Here's how the part is built. I have some questions about the finished solid (model axes, mm). Face numbers are marked on the shaded views. A direction names the side the tool comes from. Round coordinates to 2 decimals unless told otherwise and drop trailing zeros. Loops run counter-clockwise (first coordinate to the right, second up) from the corner with the lowest first, then second, coordinate; pieces in that order, holes last. Notation, with made-up numbers: M 45,-29.75 L 101,-29.75 A25 ccw 101,7.25 Z; hole C 2,9.25 d8. An arc over 180 degrees is marked long. Answer as a JSON object with one key per item and string values.
Solid Edge part; units mm, degrees
sketch "Sketch1" plane through (0, 0, 0) normal (0, -1, 0) x (1, 0, 0)
  line L0 (38.1517, 0) -> (38.1517, -10)
  line L1 (38.1517, -10) -> (28.1517, -10)
  line L2 (28.1517, -10) -> (28.1517, -20)
  line L3 (28.1517, -20) -> (38.1517, -20)
  line L4 (38.1517, -20) -> (38.1517, -46)
  line L5 (38.1517, -46) -> (28.1517, -46)
  line L6 (28.1517, -46) -> (28.1517, -56)
  line L7 (-21.8483, -56) -> (28.1517, -56)
  line L8 (-21.8483, -46) -> (-21.8483, -56)
  line L9 (-31.8483, -46) -> (-21.8483, -46)
  line L10 (-31.8483, -20) -> (-31.8483, -46)
  line L11 (-21.8483, -20) -> (-31.8483, -20)
  line L12 (-21.8483, -10) -> (-21.8483, -20)
  line L13 (-31.8483, -10) -> (-21.8483, -10)
  line L14 (-31.8483, 0) -> (-31.8483, -10)
  line L15 (-36.8483, 0) -> (-31.8483, 0)
  line L16 (-36.8483, 37) -> (-36.8483, 0)
  line L17 (-36.8483, 37) -> (43.1517, 37)
  line L18 (43.1517, 37) -> (43.1517, 0)
  line L19 (38.1517, 0) -> (43.1517, 0)
extrude "Extrusionsausprägung_1" add sketch "Sketch1" against normal blind 5 and the other way blind 0.001
sketch "Sketch2" plane through (3.1517, 5, -9.5) normal (0, 1, 0) x (0, 0, -1)
  line L0 (-46.5, 40) -> (-22.5, 40)
  line L1 (-22.5, 40) -> (-22.5, -40)
  line L2 (-22.5, -40) -> (-48.5, -40)
  line L3 (-48.5, -40) -> (-48.5, 40)
  line L4 (-48.5, 40) -> (-46.5, 40)
extrude "Extrusionsausprägung_2" add sketch "Sketch2" along normal blind 5 and the other way blind 0.001
sketch "Sketch3" plane through (43.1517, 4.9995, 19.5) normal (1, 0, 0) x (0, 0, -1)
  line L0 (-19.5, 5.0005) -> (6.5, 0.0005)
  line L1 (6.5, 0.0005) -> (9.9801, 7.8832)
  line L2 (9.9801, 7.8832) -> (-19.5, 5.0005)
extrude "Extrusionsausschnitt_1" cut sketch "Sketch3" against normal blind 96.3179
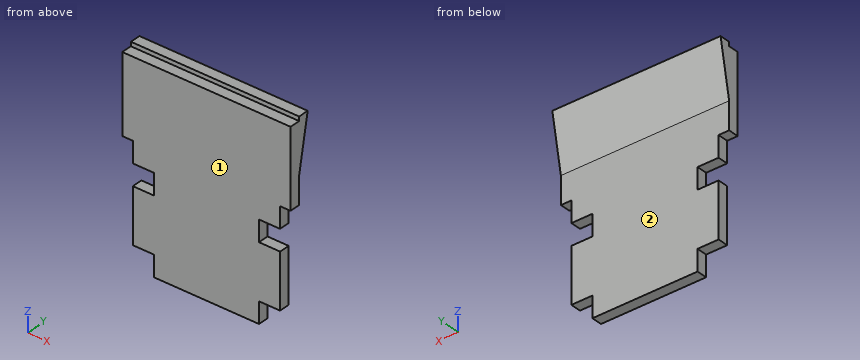
Item 1: I want a section at A-A on x = 32. List the corners of the cut face in (y, z) for me, plus the area to 3 significant figures.
Solution:
{"outline": "M 0,-46 L 5,-46 L 5,-20 L 0,-20 Z; M 0,-10 L 5,-10 L 5,13 L 10,39 L 5,39 L 5,37 L 0,37 Z", "area": "430 mm2"}
Item 2: For P1, Ø2.5, axis at x = -27, y = 3.5, coming from the -Z side; P2, Ø1.5, axis at x = 20, y = 3, coming from the +Z side; P3, Ø1.5, axis at y = 3, z = -17, coming from the +X side; P4, Ø5.5, axis at x = 32.5, y = 3.5, coming from the +Z side, each with a flat end and sliding along its axis, tell me the tip position at first contact or that it passes through.
Solution:
{"P1": "stops at z = -46", "P2": "stops at z = 37", "P3": "stops at x = 28.15", "P4": "stops at z = 39"}
Item 3: I want a section at C-C on x = 16. List the corners of the cut face in (y, z) for me, plus the area to 3 significant figures.
Solution:
{"outline": "M 0,-56 L 5,-56 L 5,13 L 10,39 L 5,39 L 5,37 L 0,37 Z", "area": "530 mm2"}
Item 4: I want a section at D-D on z = -32. List the corners of the cut face in (x, y) for me.
Solution:
{"outline": "M -31.85,0 L 38.15,0 L 38.15,5 L -31.85,5 Z"}
Item 5: For the marked faces 1 and 2, which set-ups out of +Z, -Z, +X, -X, +Y, -Y let a thin tool reach every point of the face, with its end or its side?
Solution:
{"face 1": "+Z, -Z, +X, -X, -Y", "face 2": "-Z, +X, -X, +Y"}
Item 6: If I drill on L1, parallel to Z at x = 32, y = 4.5; L2, parallel to Y at x = -6, z = -26; L3, parallel to Z at x = 10.5, y = 2.75, over which ranges is the centre line in solid material (lowest first)? Write a range as from..to.
Solution:
{"L1": "z = -46..-20, -10..37", "L2": "y = 0..5", "L3": "z = -56..37"}
Item 7: I want a section at B-B on y = 3.5. List the corners of the cut face in (x, z) for me.
Solution:
{"outline": "M -36.85,0 L -31.85,0 L -31.85,-10 L -21.85,-10 L -21.85,-20 L -31.85,-20 L -31.85,-46 L -21.85,-46 L -21.85,-56 L 28.15,-56 L 28.15,-46 L 38.15,-46 L 38.15,-20 L 28.15,-20 L 28.15,-10 L 38.15,-10 L 38.15,0 L 43.15,0 L 43.15,37 L -36.85,37 Z"}
